Job drawing, mm, ordinate dimensions from the low corner. One solid piece. Round coordinates to 2 decimals unless told otherwise and drop trailing zeros. Order: outer loops, then holes, each group sorted by start corner. A loop starts at its lowest first (then second) coordinate and runs counter-clockwise, first axis right, second up. Notation, with made-up numbers: (60.5, 67) -> (91.5, 67) arc R21 ccw to (91.5, 80) -> close; hole circle Ø9 at (59, 28). An arc over 180 degrees is marked (long way). Use CSV: the item, a comma, the result in double quotes.
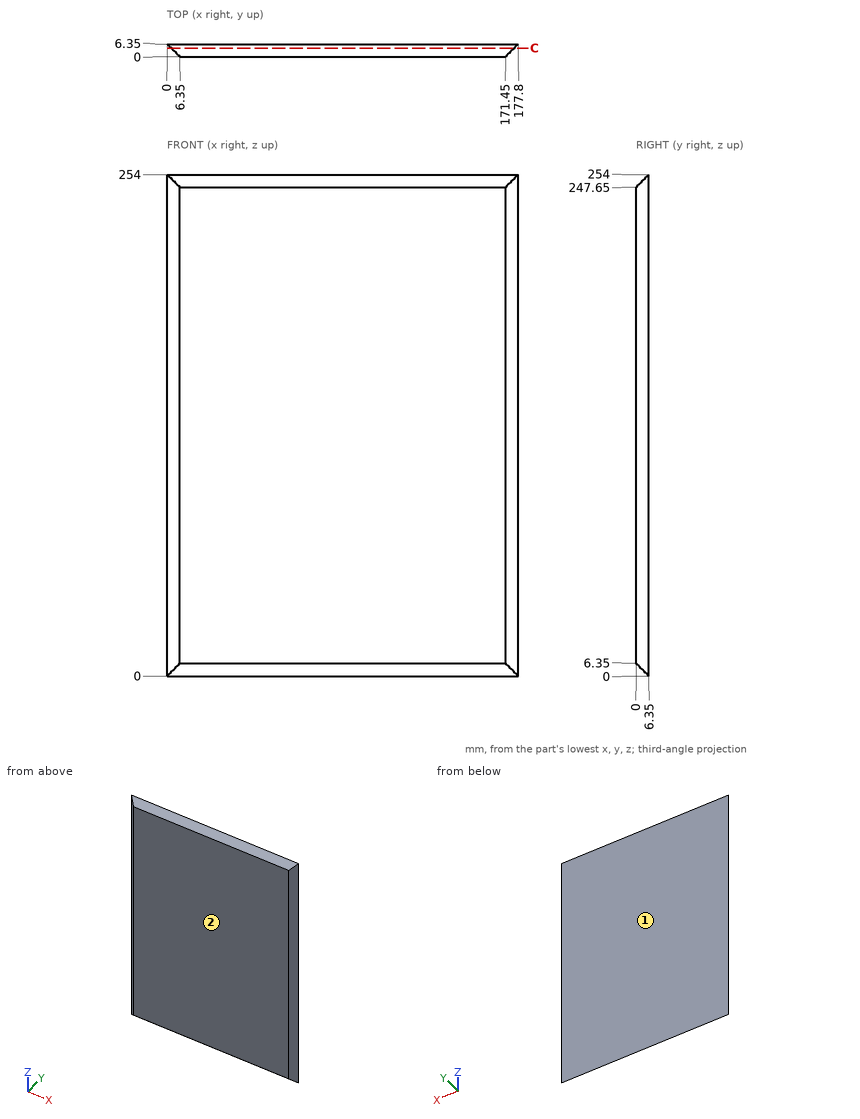
(1) Cut at C-C, the plane y = 4.25. Give the cut face in (x, z).
Reply:
outline,"(2.1, 2.1) -> (175.7, 2.1) -> (175.7, 251.9) -> (2.1, 251.9) -> close"
(2) Pull direction Y, two halves, no side cores. Call the marked faces 1 and 2: released by +Y, released by -Y, zero draft, split by the parting line, or undercut.
Reply:
face 1,"released by +Y"
face 2,"released by -Y"
(3) Probe probe 1 along X at (y, z) = (0.75, 150); probe 2 along Z at (x, y) = (129, 3.75); probe 3 along X at (y, z) = (3.5, 93). List the from-to ranges inside material, lowest first. Write a range as [from, to].
Reply:
probe 1,"[5.6, 172.2]"
probe 2,"[2.6, 251.4]"
probe 3,"[2.85, 174.95]"
(4) Drop flat-ended pins along their axis: P1, Ø1.5, axis at y = 5, z = 208.5, coming from the -X side; P2, Ø1, axis at x = 146.5, y = 4.5, coming from the -Z side. Give the stop position or say it passes through.
Reply:
P1,"x = 0.6"
P2,"z = 1.35"
